Read the model definition and answer for the solid it produces. Units are mm, in the model's axes. A direction names the side the tool comes from. Give positions to 0.01 mm unless a question says otherwise; leave off trailing zeros. Order: outer loops, then holes, each group sorted by start corner. A loop starts at its lowest first (then second) coordinate and runs counter-clockwise, first axis right, second up.
```python
from build123d import *

# Parameters (mm, degrees)
BOSS_EXTRUDE1_DEPTH = 20
SKETCH2_R           = 2.05
CUT_EXTRUDE1_DEPTH  = 88.749643874
SKETCH3_R           = 2.375
CUT_EXTRUDE2_DEPTH  = 100.121138008
FILLET1_R           = 10
FILLET2_R           = 5
FILLET3_R           = 2


with BuildPart() as part:
    # Sketch1 → Boss-Extrude1 (new body)
    with BuildSketch(Plane(origin=(0, 0, 0), x_dir=(1, 0, 0), z_dir=(0, 1, 0))):
        Polygon((0, 0), (-5, 0), (-5, -25), (30, -25), (30, -0.579896907), (30, 25), (80, 25), (80, 30), (25, 30), (25, -20), (0, -20), align=None)
    extrude(amount=BOSS_EXTRUDE1_DEPTH)

    # Sketch2 → Cut-Extrude1 (cut, through all)
    with BuildSketch(Plane(origin=(0, 0, 0), x_dir=(0, 0, -1), z_dir=(1, 0, 0))):
        with Locations((-10, 10)):
            Circle(SKETCH2_R)
    extrude(amount=-CUT_EXTRUDE1_DEPTH, mode=Mode.SUBTRACT)

    # Sketch3 → Cut-Extrude2 (cut, through all)
    with BuildSketch(Plane(origin=(0, 0, -30), x_dir=(-1, 0, 0), z_dir=(0, 0, -1))):
        with Locations((-68, 10)):
            Circle(SKETCH3_R)
        with Locations((-44, 10)):
            Circle(SKETCH3_R)
    extrude(amount=-CUT_EXTRUDE2_DEPTH, mode=Mode.SUBTRACT)

    # Fillet1
    fillet1_edges = [part.edges().sort_by_distance(p)[0] for p in [
        (30, 10, -25),
    ]]
    fillet(fillet1_edges, radius=FILLET1_R)

    # Fillet2
    fillet2_edges = [part.edges().sort_by_distance(p)[0] for p in [
        (25, 10, -30),
        (30, 10, 25),
        (-5, 10, 25),
    ]]
    fillet(fillet2_edges, radius=FILLET2_R)

    # Fillet3
    fillet3_edges = [part.edges().sort_by_distance(p)[0] for p in [
        (0, 10, 20),
        (25, 10, 20),
        (80, 10, -30),
        (80, 10, -25),
        (0, 10, 0),
    ]]
    fillet(fillet3_edges, radius=FILLET3_R)


solid = part.part
```
1) The part is cut by section B-B on z = 10. Determine the outline of the cut face in (x, y), and give its area (4 significant figures).
Final values:
outline: (-5, 0) - (0, 0) - (0, 7.95) - (-5, 7.95) - close; (-5, 12.05) - (0, 12.05) - (0, 20) - (-5, 20) - close; (25, 0) - (30, 0) - (30, 20) - (25, 20) - close
area: 179.5 mm2
2) The part is cut by section C-C on x = 44. Determine the outline of the cut face in (y, z) (3 decimals), and give its area (4 significant figures).
Final values:
outline: (0, -30) - (7.625, -30) - (7.625, -25) - (0, -25) - close; (12.375, -30) - (20, -30) - (20, -25) - (12.375, -25) - close
area: 76.25 mm2
3) A tool of negligible diameter and unlimited length cuts with its end or side. For faces 4 (the face through (-0.6, 10.14, 0.57)), 5 (the face through (41.735, 10.713, -27.535)), 6 (the face through (30, 10, 3)), 7 (the face through (-2.465, 8.753, 11.627)), from which of +Z, -Z, +X, -X, +Y, -Y can it reach the whole face along a straight path? Write none if from no direction.
Final values:
face 4: -Z, +Y, -Y
face 5: +Z, -Z
face 6: +Z, +X, +Y, -Y
face 7: -X
4) Given pin 1 (4.5 mm diameter, centred on x = 68, y = 10, fed in from -Z); pin 2 (10 mm diameter, centred on x = 62, y = 14, fed in from +Z); pin 3 (3.5 mm diameter, centred on y = 10, z = 10, fed in from +X); pin 4 (2.5 mm diameter, centred on x = -3, y = 9, fed in from -Z), each flat-ended and moving along its own axis, determine where each tip first touches the part or whether it passes through.
Final values:
pin 1: passes through
pin 2: stops at z = -25
pin 3: stops at x = 30
pin 4: stops at z = 0
5) For a pull along Y with two mould halves and no side action, classify faces 1 (the face through (28, 20, -5)), 2 (the face through (-5, 7.6, 9.9)), 3 (the face through (65.735, 10.713, -27.535)) as released by +Y, released by -Y, zero draft, split by the parting line, or undercut.
Final values:
face 1: released by +Y
face 2: zero draft
face 3: undercut
6) The part is cut by section D-D on z = 16. Determine the outline of the cut face in (x, y).
Final values:
outline: (-5, 0) - (0, 0) - (0, 20) - (-5, 20) - close; (25, 0) - (30, 0) - (30, 20) - (25, 20) - close
7) The part is cut by section A-A on y = 10. Count the separate pieces of the cut face and the enclosed holes in it, and give its area (3 significant figures).
Final values:
separate pieces: 4
enclosed holes: 0
area: 712 mm2
8) Consider L1, parallel to Y at x = 68, z = -26.25 (3 decimals); L2, parallel to X at y = 1.5, z = 13.5; L3, parallel to Y at x = -2.95, z = 10. Determine where each line is inside the solid, lowest interval first.
Final values:
L1: y = 0 to 7.625, 12.375 to 20
L2: x = -5 to 0, 25 to 30
L3: y = 0 to 7.95, 12.05 to 20
